Check sheet for the modelled part. Datum: model origin and axes. Units: mm. Face numbers are marked on the shaded views. A direction names the side the tool comes from. Coordinates: 2 decimals unless noted, no trailing zeros. Write each loop counter-clockwise with the first axis right and the second up, starting at its lowest first coordinate (ties: lowest second). Pieces come first, ordered by that corner, then holes. Notation, with made-up numbers: (-10, -32) - (33, -32) arc R27 ccw to (33, 1) - close; hole circle Ø10 at (41.5, 67.25). An arc over 180 degrees is marked (long way). Write each question's results on one line, items separated by ' | '.
from build123d import *

# Parameters (mm, degrees)
SKETCH1_W           = 100
SKETCH1_H           = 100
BOSS_EXTRUDE2_DEPTH = 40
SKETCH3_W           = 20
SKETCH3_H           = 10
CUT_EXTRUDE3_DEPTH  = 100
SKETCH4_R           = 29.179887526
CUT_EXTRUDE5_DEPTH  = 100
SKETCH5_W           = 60
SKETCH5_H           = 20
CUT_EXTRUDE6_DEPTH  = 100
SKETCH6_W           = 22
SKETCH6_H           = 32
CUT_EXTRUDE7_DEPTH  = 15
SKETCH7_W           = 22
SKETCH7_H           = 10
CUT_EXTRUDE9_DEPTH  = 100
SKETCH9_W           = 32
SKETCH9_H           = 22
CUT_EXTRUDE10_DEPTH = 15
SKETCH10_W          = 32
SKETCH10_H          = 22
CUT_EXTRUDE11_DEPTH = 15
SKETCH11_W          = 33
SKETCH11_H          = 33
CUT_EXTRUDE13_DEPTH = 22
SKETCH12_W          = 33
SKETCH12_H          = 33
CUT_EXTRUDE14_DEPTH = 22
SKETCH13_W          = 30
SKETCH13_H          = 20
CUT_EXTRUDE15_DEPTH = 100
SKETCH14_W          = 12
SKETCH14_H          = 16
CUT_EXTRUDE17_DEPTH = 80
SKETCH15_W          = 24
SKETCH15_H          = 52
CUT_EXTRUDE18_DEPTH = 15
SKETCH16_W          = 30
SKETCH16_H          = 44.18
CUT_EXTRUDE19_DEPTH = 15
SKETCH17_W          = 11
SKETCH17_H          = 26
CUT_EXTRUDE20_DEPTH = 15
SKETCH18_W          = 11
SKETCH18_H          = 26
CUT_EXTRUDE22_DEPTH = 15
SKETCH19_W          = 11
SKETCH19_H          = 17
CUT_EXTRUDE26_DEPTH = 2.2
SKETCH20_R          = 2.5
CUT_EXTRUDE32_DEPTH = 17
SKETCH21_W          = 4
SKETCH21_H          = 12
CUT_EXTRUDE33_DEPTH = 4
SKETCH23_W          = 11
SKETCH23_H          = 17
CUT_EXTRUDE34_DEPTH = 2.2
SKETCH24_R          = 2.5
CUT_EXTRUDE35_DEPTH = 17
SKETCH25_W          = 4
SKETCH25_H          = 12
CUT_EXTRUDE36_DEPTH = 3
SKETCH26_R          = 3
CUT_EXTRUDE37_DEPTH = 3
SKETCH27_R          = 3
CUT_EXTRUDE38_DEPTH = 3
SKETCH28_W          = 17
SKETCH28_H          = 11
CUT_EXTRUDE39_DEPTH = 2.2
SKETCH29_R          = 3
CUT_EXTRUDE40_DEPTH = 4
SKETCH30_W          = 4
SKETCH30_H          = 4.8
CUT_EXTRUDE43_DEPTH = 7
SKETCH31_W          = 4
SKETCH31_H          = 4.8
CUT_EXTRUDE44_DEPTH = 7
CUT_EXTRUDE45_DEPTH = 100
SKETCH34_W          = 5
SKETCH34_H          = 20
CUT_EXTRUDE46_DEPTH = 100
CUT_EXTRUDE47_DEPTH = 100
SKETCH36_W          = 5.5
SKETCH36_H          = 15.404877169
BOSS_EXTRUDE3_DEPTH = 55
SKETCH37_W          = 20.232210009
SKETCH37_H          = 11
CUT_EXTRUDE48_DEPTH = 3
SKETCH38_W          = 40
SKETCH38_H          = 86
CUT_EXTRUDE53_DEPTH = 1


with BuildPart() as part:
    # Sketch1 → Boss-Extrude2 (new body)
    with BuildSketch(Plane(origin=(0, 0, 0), x_dir=(1, 0, 0), z_dir=(0, 1, 0))):
        Rectangle(SKETCH1_W, SKETCH1_H)
    extrude(amount=BOSS_EXTRUDE2_DEPTH)

    # Sketch3 → Cut-Extrude3 (cut)
    with BuildSketch(Plane(origin=(50, 0, 0), x_dir=(0, 0, -1), z_dir=(1, 0, 0))):
        with Locations((-1.010205144, 10)):
            Rectangle(SKETCH3_W, SKETCH3_H)
    extrude(amount=-CUT_EXTRUDE3_DEPTH, mode=Mode.SUBTRACT)

    # Sketch4 → Cut-Extrude5 (cut)
    with BuildSketch(Plane.XY.offset(50)):
        with Locations((63.191438408, 23.747323898)):
            Circle(SKETCH4_R)
    extrude(amount=-CUT_EXTRUDE5_DEPTH, mode=Mode.SUBTRACT)

    # Sketch5 → Cut-Extrude6 (cut)
    with BuildSketch(Plane.XY.offset(50)):
        with Locations((8.956827713, 30)):
            Rectangle(SKETCH5_W, SKETCH5_H)
    extrude(amount=-CUT_EXTRUDE6_DEPTH, mode=Mode.SUBTRACT)

    # Sketch6 → Cut-Extrude7 (cut)
    with BuildSketch(Plane(origin=(0, 20, 0), x_dir=(1, 0, 0), z_dir=(0, 1, 0))):
        with Locations((23.190442589, 0)):
            Rectangle(SKETCH6_W, SKETCH6_H)
    extrude(amount=-CUT_EXTRUDE7_DEPTH, mode=Mode.SUBTRACT)

    # Sketch7 → Cut-Extrude9 (cut)
    with BuildSketch(Plane.XY.offset(50)):
        with Locations((13.743053617, 10)):
            Rectangle(SKETCH7_W, SKETCH7_H)
    extrude(amount=-CUT_EXTRUDE9_DEPTH, mode=Mode.SUBTRACT)

    # Sketch9 → Cut-Extrude10 (cut)
    with BuildSketch(Plane(origin=(0, 20, 0), x_dir=(1, 0, 0), z_dir=(0, 1, 0))):
        with Locations((13.743053617, -34.588860887)):
            Rectangle(SKETCH9_W, SKETCH9_H)
    extrude(amount=-CUT_EXTRUDE10_DEPTH, mode=Mode.SUBTRACT)

    # Sketch10 → Cut-Extrude11 (cut)
    with BuildSketch(Plane(origin=(0, 20, 0), x_dir=(1, 0, 0), z_dir=(0, 1, 0))):
        with Locations((13.743053617, 34.59)):
            Rectangle(SKETCH10_W, SKETCH10_H)
    extrude(amount=-CUT_EXTRUDE11_DEPTH, mode=Mode.SUBTRACT)

    # Sketch11 → Cut-Extrude13 (cut)
    with BuildSketch(Plane.XY.offset(50)):
        with Locations((-33.5, 16.5)):
            Rectangle(SKETCH11_W, SKETCH11_H)
    extrude(amount=-CUT_EXTRUDE13_DEPTH, mode=Mode.SUBTRACT)

    # Sketch12 → Cut-Extrude14 (cut)
    with BuildSketch(Plane(origin=(0, 0, -50), x_dir=(-1, 0, 0), z_dir=(0, 0, -1))):
        with Locations((33.5, 16.5)):
            Rectangle(SKETCH12_W, SKETCH12_H)
    extrude(amount=-CUT_EXTRUDE14_DEPTH, mode=Mode.SUBTRACT)

    # Sketch13 → Cut-Extrude15 (cut)
    with BuildSketch(Plane(origin=(0, 0, -50), x_dir=(-1, 0, 0), z_dir=(0, 0, -1))):
        with Locations((36.043172287, 30)):
            Rectangle(SKETCH13_W, SKETCH13_H)
    extrude(amount=-CUT_EXTRUDE15_DEPTH, mode=Mode.SUBTRACT)

    # Sketch14 → Cut-Extrude17 (cut)
    with BuildSketch(Plane.XY.offset(28)):
        with Locations((-33.5, 12.595122831)):
            Rectangle(SKETCH14_W, SKETCH14_H)
    extrude(amount=-CUT_EXTRUDE17_DEPTH, mode=Mode.SUBTRACT)

    # Sketch15 → Cut-Extrude18 (cut)
    with BuildSketch(Plane(origin=(0, 20, 0), x_dir=(1, 0, 0), z_dir=(0, 1, 0))):
        with Locations((-33.5, 0)):
            Rectangle(SKETCH15_W, SKETCH15_H)
    extrude(amount=-CUT_EXTRUDE18_DEPTH, mode=Mode.SUBTRACT)

    # Sketch16 → Cut-Extrude19 (cut)
    with BuildSketch(Plane(origin=(0, 20, 0), x_dir=(1, 0, 0), z_dir=(0, 1, 0))):
        with Locations((-4.309557411, 0.001139113)):
            Rectangle(SKETCH16_W, SKETCH16_H)
    extrude(amount=-CUT_EXTRUDE19_DEPTH, mode=Mode.SUBTRACT)

    # Sketch17 → Cut-Extrude20 (cut)
    with BuildSketch(Plane(origin=(0, 20, 0), x_dir=(1, 0, 0), z_dir=(0, 1, 0))):
        with Locations((-9.626946383, 34.59)):
            Rectangle(SKETCH17_W, SKETCH17_H)
    extrude(amount=-CUT_EXTRUDE20_DEPTH, mode=Mode.SUBTRACT)

    # Sketch18 → Cut-Extrude22 (cut)
    with BuildSketch(Plane(origin=(0, 20, 0), x_dir=(1, 0, 0), z_dir=(0, 1, 0))):
        with Locations((-9.63, -34.691148393)):
            Rectangle(SKETCH18_W, SKETCH18_H)
    extrude(amount=-CUT_EXTRUDE22_DEPTH, mode=Mode.SUBTRACT)

    # Sketch19 → Cut-Extrude26 (cut)
    with BuildSketch(Plane(origin=(0, 0, 0), x_dir=(-1, 0, 0), z_dir=(0, -1, 0))):
        with Locations((-37.734715737, -36.5)):
            Rectangle(SKETCH19_W, SKETCH19_H)
    extrude(amount=-CUT_EXTRUDE26_DEPTH, mode=Mode.SUBTRACT)

    # Sketch20 → Cut-Extrude32 (cut)
    with BuildSketch(Plane(origin=(0, 0, 0), x_dir=(-1, 0, 0), z_dir=(0, -1, 0))):
        with Locations((-32.234715737, -45)):
            Circle(SKETCH20_R)
    extrude(amount=-CUT_EXTRUDE32_DEPTH, mode=Mode.SUBTRACT)

    # Sketch21 → Cut-Extrude33 (cut)
    with BuildSketch(Plane.ZY.offset(-29.743053617)):
        with Locations((44.433350435, 14)):
            Rectangle(SKETCH21_W, SKETCH21_H)
    extrude(amount=-CUT_EXTRUDE33_DEPTH, mode=Mode.SUBTRACT)

    # Sketch23 → Cut-Extrude34 (cut)
    with BuildSketch(Plane(origin=(0, 0, 0), x_dir=(-1, 0, 0), z_dir=(0, -1, 0))):
        with Locations((-37.734715737, 36.5)):
            Rectangle(SKETCH23_W, SKETCH23_H)
    extrude(amount=-CUT_EXTRUDE34_DEPTH, mode=Mode.SUBTRACT)

    # Sketch24 → Cut-Extrude35 (cut)
    with BuildSketch(Plane.XZ):
        with Locations((32.234715737, -45)):
            Circle(SKETCH24_R)
    extrude(amount=-CUT_EXTRUDE35_DEPTH, mode=Mode.SUBTRACT)

    # Sketch25 → Cut-Extrude36 (cut)
    with BuildSketch(Plane.ZY.offset(-29.743053617)):
        with Locations((-43.59, 14)):
            Rectangle(SKETCH25_W, SKETCH25_H)
    extrude(amount=-CUT_EXTRUDE36_DEPTH, mode=Mode.SUBTRACT)

    # Sketch26 → Cut-Extrude37 (cut)
    with BuildSketch(Plane(origin=(-2.256946383, 0, 0), x_dir=(0, 0, -1), z_dir=(1, 0, 0))):
        with Locations((-28.588860887, 12)):
            Circle(SKETCH26_R)
    extrude(amount=-CUT_EXTRUDE37_DEPTH, mode=Mode.SUBTRACT)

    # Sketch27 → Cut-Extrude38 (cut)
    with BuildSketch(Plane(origin=(-2.256946383, 0, 0), x_dir=(0, 0, -1), z_dir=(1, 0, 0))):
        with Locations((28.59, 12)):
            Circle(SKETCH27_R)
    extrude(amount=-CUT_EXTRUDE38_DEPTH, mode=Mode.SUBTRACT)

    # Sketch28 → Cut-Extrude39 (cut)
    with BuildSketch(Plane.XZ):
        with Locations((-40.055873336, 0)):
            Rectangle(SKETCH28_W, SKETCH28_H)
    extrude(amount=-CUT_EXTRUDE39_DEPTH, mode=Mode.SUBTRACT)

    # Sketch29 → Cut-Extrude40 (cut)
    with BuildSketch(Plane(origin=(0, 2.2, 0), x_dir=(-1, 0, 0), z_dir=(0, -1, 0))):
        with Locations((47.799920192, -0.070169229)):
            Circle(SKETCH29_R)
    extrude(amount=-CUT_EXTRUDE40_DEPTH, mode=Mode.SUBTRACT)

    # Sketch30 → Cut-Extrude43 (cut)
    with BuildSketch(Plane.XY.offset(-22.091139113)):
        with Locations((-2.126946383, 11.349361099)):
            Rectangle(SKETCH30_W, SKETCH30_H)
    extrude(amount=-CUT_EXTRUDE43_DEPTH, mode=Mode.SUBTRACT)

    # Sketch31 → Cut-Extrude44 (cut)
    with BuildSketch(Plane(origin=(0, 0, 22.088860887), x_dir=(-1, 0, 0), z_dir=(0, 0, -1))):
        with Locations((2.13, 11.35)):
            Rectangle(SKETCH31_W, SKETCH31_H)
    extrude(amount=-CUT_EXTRUDE44_DEPTH, mode=Mode.SUBTRACT)

    # Sketch33 → Cut-Extrude45 (cut)
    with BuildSketch(Plane(origin=(0, 0, -28), x_dir=(-1, 0, 0), z_dir=(0, 0, -1))):
        Polygon((45, 0), (50, 5), (50, 0), align=None)
    extrude(amount=-CUT_EXTRUDE45_DEPTH, mode=Mode.SUBTRACT)

    # Sketch34 → Cut-Extrude46 (cut)
    with BuildSketch(Plane.XY.offset(28)):
        with Locations((-47.5, 10)):
            Rectangle(SKETCH34_W, SKETCH34_H)
    extrude(amount=-CUT_EXTRUDE46_DEPTH, mode=Mode.SUBTRACT)

    # Sketch35 → Cut-Extrude47 (cut)
    with BuildSketch(Plane.XY.offset(28)):
        Polygon((-45, 4.595122831), (-39.5, 0), (-45, 0), align=None)
    extrude(amount=-CUT_EXTRUDE47_DEPTH, mode=Mode.SUBTRACT)

    # Sketch36 → Boss-Extrude3 (add)
    with BuildSketch(Plane.XY.offset(28)):
        with Locations((-42.25, 12.297561416)):
            Rectangle(SKETCH36_W, SKETCH36_H)
    extrude(amount=-BOSS_EXTRUDE3_DEPTH)

    # Sketch37 → Cut-Extrude48 (cut)
    with BuildSketch(Plane(origin=(0, 0, 0), x_dir=(-1, 0, 0), z_dir=(0, -1, 0))):
        with Locations((32.017121667, 0)):
            Rectangle(SKETCH37_W, SKETCH37_H)
    extrude(amount=-CUT_EXTRUDE48_DEPTH, mode=Mode.SUBTRACT)

    # Sketch38 → Cut-Extrude53 (cut)
    with BuildSketch(Plane(origin=(0, 3, 0), x_dir=(-1, 0, 0), z_dir=(0, -1, 0))):
        with Locations((-6.777878387, 0)):
            Rectangle(SKETCH38_W, SKETCH38_H)
    extrude(amount=-CUT_EXTRUDE53_DEPTH, mode=Mode.SUBTRACT)


solid = part.part
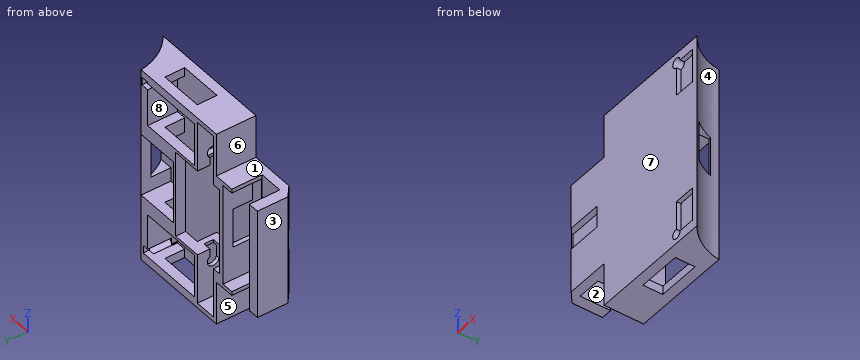
1. Go/stop test with flat-tipped pins: pin 1 (1 mm diameter, centred on x = -14, z = 31, fed in from -Y); pin 2 (5.5 mm diameter, centred on x = 38, z = 32.5, fed in from -Y); pin 3 (4.5 mm diameter, centred on y = 10, z = 36.5, fed in from -X); pin 4 (12 mm diameter, centred on y = 7.5, z = -19, fed in from +X). Record where each tip stops, or that it passes through.
Values follow:
pin 1: stops at y = 0 | pin 2: stops at y = 2.2 | pin 3: stops at x = -17 | pin 4: stops at x = 44.31
2. Sectioned sample at C-C (y = 18.5). Give the number of separate pieces and of enclosed holes in the cut face, then the cut area to 3 significant figures.
Values follow:
separate pieces: 2 | enclosed holes: 4 | area: 1,710 mm^2
3. Material ranges on L1, parallel to Z at x = 29, y = 19; L2, parallel to Y at x = -2.9, z = -28.59; L3, parallel to Y at x = -1, z = -25, recorded low to high. Write a range as [from, to].
Values follow:
L1: z = [-50, -45.59], [-23.59, -16], [16, 23.59], [45.59, 50] | L2: y = [0, 3], [4, 8.95], [15, 20] | L3: y = [0, 3], [4, 5]
4. Access from +Z, -Z, +X, -X, +Y, -Y to the whole of each face (thin tool, end or side, straight path). Record for the marked faces 4, 5, 6, 7 and 8.
Values follow:
face 4: +Z, -Z, +X, +Y | face 5: -Z, -X, +Y, -Y | face 6: +Z, -X, +Y, -Y | face 7: +Z, -Z, +X, -X, -Y | face 8: +Y
5. Sectioned sample at B-B (z = 19). Record the cut outline in (x, y), then the cut area to 3 significant figures.
Values follow:
outline: (-45, 4.6) - (-39.5, 0) - (46.23, 0) arc R29.18 cw to (34.25, 20) - (10.69, 20) - (10.69, 15) - (24.74, 15) - (24.74, 5) - (-19.31, 5) - (-19.31, 20) - (-21.5, 20) - (-21.5, 5) - (-27.5, 5) - (-27.5, 4.6) - (-39.5, 4.6) - (-39.5, 20) - (-45, 20) - close; hole (-13.22, 3) - (26.78, 3) - (26.78, 4) - (-13.22, 4) - close | area: 749 mm^2
6. Sectioned sample at A-A (x = 7.5). Record the cut outline in (y, z).
Values follow:
outline: (0, -50) - (5, -50) - (5, 50) - (0, 50) - close; (15, -50) - (20, -50) - (20, -45.59) - (15, -45.59) - close; (15, -23.59) - (20, -23.59) - (20, -22.09) - (15, -22.09) - close; (15, 22.09) - (20, 22.09) - (20, 23.59) - (15, 23.59) - close; (15, 45.59) - (20, 45.59) - (20, 50) - (15, 50) - close; hole (3, -43) - (4, -43) - (4, 43) - (3, 43) - close
7. Draft check along X on the marked faces 1, 2 and 3. Enter one of: pulls with the +X half, pulls with the -X half, needs draft (parallel to the pull), parting line crosses it, or undercut.
Values follow:
face 1: needs draft | face 2: undercut | face 3: pulls with the -X half
8. Sectioned sample at D-D (x = 28.5). Record the cut outline in (y, z), then the cut area to 3 significant figures.
Values follow:
outline: (0, -50) - (20, -50) - (20, -45.59) - (5, -45.59) - (5, -23.59) - (20, -23.59) - (20, -16) - (5, -16) - (5, 16) - (20, 16) - (20, 23.59) - (5, 23.59) - (5, 45.59) - (20, 45.59) - (20, 50) - (0, 50) - close | area: 860 mm^2
